from build123d import *

# Parameters (mm, degrees)
SKETCH1_R           = 3
BOSS_EXTRUDE1_DEPTH = 3
SKETCH2_R           = 1.25
CUT_EXTRUDE1_DEPTH  = 6.196152423
FILLET1_R           = 0.3
SKETCH3_W           = 1
SKETCH3_H           = 8
CUT_EXTRUDE3_DEPTH  = 1


with BuildPart() as part:
    # Sketch1 → Boss-Extrude1 (new body)
    with BuildSketch(Plane.XY):
        Circle(SKETCH1_R)
    extrude(amount=BOSS_EXTRUDE1_DEPTH)

    # Sketch2 → Cut-Extrude1 (cut, through all)
    with BuildSketch(Plane.XY.offset(3)):
        Circle(SKETCH2_R)
    extrude(amount=-CUT_EXTRUDE1_DEPTH, mode=Mode.SUBTRACT)

    # Fillet1
    fillet1_edges = [part.edges().sort_by_distance(p)[0] for p in [
        (-3, 0, 3),
        (-1.25, 0, 0),
        (-1.25, 0, 3),
    ]]
    fillet(fillet1_edges, radius=FILLET1_R)

    # Sketch3 → Cut-Extrude3 (cut)
    with BuildSketch(Plane.XY.offset(3)):
        Rectangle(SKETCH3_W, SKETCH3_H)
    extrude(amount=-CUT_EXTRUDE3_DEPTH, mode=Mode.SUBTRACT)


solid = part.part
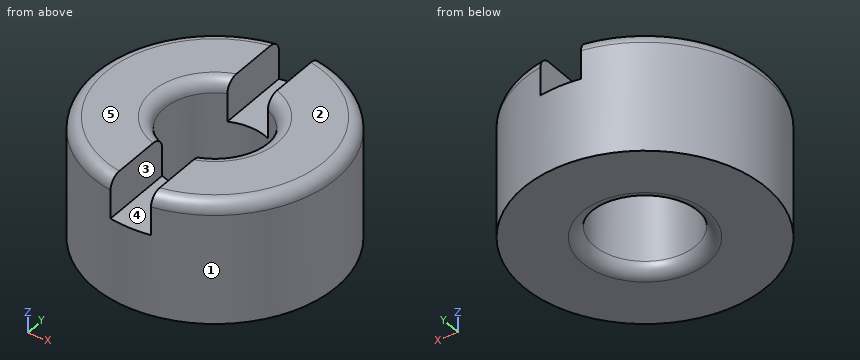
Work out the finished part from the listing and answer in its coordinate system (mm). Face numbers are marked on the shaded views. A direction names the side the tool comes from. Round coordinates to 2 decimals unless told otherwise and drop trailing zeros. Write each loop counter-clockwise with the first axis right and the second up, starting at its lowest first coordinate (ties: lowest second). Pieces come first, ordered by that corner, then holes. Notation, with made-up numbers: (80.5, 37) - (126.5, 37) arc R19 cw to (126.5, 57) - close; hole circle Ø5 at (-26, 46.25). An arc over 180 degrees is marked (long way). Answer in a Markdown table with one row per item. Add a question column.
1. For the marked faces 4 and 5, determine the directions among +Z, -Z, +X, -X, +Y, -Y from which every point of the face is accessible in a straight line to the end or side of a thin tool.
2. A cutting plane is placed at A-A, the plane x = 0. Determine the outline of the cut face in (y, z).
3. The mould has two halves that part along X. Classify the marked faces 1, 2 and 3: +X half, -X half, draft (parallel to the pull), parting line (faces both ways), or undercut.
4. A cutting plane is placed at B-B, the plane y = 0. Determine the outline of the cut face in (x, z), and give its area (3 significant figures).
5. Given pin 1 (1.1 mm diameter, centred on y = 2, z = 2.5, fed in from -X); pin 2 (1.5 mm diameter, centred on x = -2, z = 2.5, fed in from -Y); pin 3 (2 mm diameter, centred on x = -2, y = 2, fed in from -Z); pin 4 (0.5 mm diameter, centred on x = 0, y = 1.5, fed in from +Z), each flat-ended and moving along its own axis, determine where each tip first touches the part or whether it passes through.
6. A cutting plane is placed at C-C, the plane z = 0.8. Determine the outline of the cut face in (x, y).
7. Find the intervals of material crossed by line 1 along Y through (x, z) = (0, 1.1); line 2 along X through (y, z) = (-0.7, 2.9), in increasing order. Write a range as from..to.
Worked out:
| question | item | result |
|---|---|---|
| 1 | face 4 | +Z, +Y, -Y |
| 1 | face 5 | +Z, +X, -X, +Y, -Y |
| 2 | outline | (-3, 0) - (-1.55, 0) arc R0.3 ccw to (-1.25, 0.3) - (-1.25, 2) - (-3, 2) - close; (1.25, 0.3) arc R0.3 ccw to (1.55, 0) - (3, 0) - (3, 2) - (1.25, 2) - close |
| 3 | face 1 | parting line |
| 3 | face 2 | draft |
| 3 | face 3 | undercut |
| 4 | outline | (-3, 0) - (-1.55, 0) arc R0.3 ccw to (-1.25, 0.3) - (-1.25, 2.7) arc R0.3 ccw to (-1.55, 3) - (-2.7, 3) arc R0.3 ccw to (-3, 2.7) - close; (1.25, 0.3) arc R0.3 ccw to (1.55, 0) - (3, 0) - (3, 2.7) arc R0.3 ccw to (2.7, 3) - (1.55, 3) arc R0.3 ccw to (1.25, 2.7) - close |
| 4 | area | 10.4 mm^2 |
| 5 | pin 1 | x = -2.63 |
| 5 | pin 2 | y = -2.73 |
| 5 | pin 3 | z = 0 |
| 5 | pin 4 | z = 2 |
| 6 | outline | circle Ø6 at (0, 0); hole circle Ø2.5 at (0, 0) |
| 7 | line 1 | -3..-1.25, 1.25..3 |
| 7 | line 2 | -2.84..-1.13, 1.13..2.84 |
